Geometry: final body of the model. Coordinates: model frame, mm. A direction names the side the tool comes from. Round coordinates to 2 decimals unless told otherwise and drop trailing zeros. Loops run counter-clockwise (first coordinate to the right, second up) from the corner with the lowest first, then second, coordinate; pieces in that order, holes last. Notation, with made-up numbers: M -19,-12 L 20,-12 A36 cw 20,26 Z; hole C 49.5,28.5 d4. An arc over 180 degrees is marked long. Answer as a JSON object with one key per item and string values.
```python
from build123d import *


with BuildPart() as part:
    # Sketch1 → Revolve1 (revolve)
    with BuildSketch(Plane(origin=(0, 0, 0), x_dir=(1, 0, 0), z_dir=(0, 1, 0))):
        with BuildLine():
            Line((0, -25.572091464), (18.57375, -25.572091464))
            Line((18.57375, -25.572091464), (18.57375, -24.046641665))
            Line((18.57375, -24.046641665), (16.684625, -22.157516665))
            add(Edge.make_bspline(
                [(16.684625, -22.157516665), (11.468108673, -19.962544079), (7.225955877, -16.564924261), (4.020652898, -12.022441155)],
                knots=[0, 0, 0, 0, 0.953211626, 0.953211626, 0.953211626, 0.953211626], degree=3))
            ThreePointArc((4.020652898, -12.022441155), (3.674948406, -11.326203905), (3.556, -10.558018263))
            Line((3.556, -10.558018263), (3.556, 20.823171826))
            Line((3.556, 20.823171826), (0, 20.823171826))
            Line((0, 20.823171826), (0, -25.572091464))
        make_face()
    revolve(axis=Axis((0, 0, 25.572091464), (0, 0, -1)))


solid = part.part
```
1) Set-up query: faces 1 (the face through (-14.74, 11.3, 24.8)), 2 (the face through (-0.77, 3.47, -5.35)). Return all of +Z, -Z, +X, -X, +Y, -Y with unobstructed straight access to the full face (end or side cutting, diameter ignored); none if empty.
Geometry results:
{"face 1": "+Z, -Z", "face 2": "-Z"}
2) Line query: probe 1 along X at (y, z) = (-1.5, 3); probe 2 along Z at (x, y) = (-1.5, 5); probe 3 along Z at (x, y) = (12.5, -4.5). Output: solid intervals per line, ascending.
Geometry results:
{"probe 1": "-3.22 to 3.22", "probe 2": "13.61 to 25.57", "probe 3": "20.48 to 25.57"}
3) Cut plane A-A on z = -6.5. Return the cut outline in (x, y), and give its area (3 significant figures).
Geometry results:
{"outline": "C 0,0 d7.11", "area": "39.7 mm2"}
4) First-contact query: pin 1 (1.5 mm diameter, centred on x = 5.5, z = 14.5, fed in from +Y); pin 2 (10 mm diameter, centred on x = -8, z = 15.5, fed in from +Y); pin 3 (12 mm diameter, centred on x = -12.5, y = -5.5, fed in from -Z). Flat tips, straight axial feed; report the tip coordinate or a pass-through.
Geometry results:
{"pin 1": "y = 4.11", "pin 2": "y = 11.18", "pin 3": "z = 16.27"}
